```python
from build123d import *

# Parameters (mm, degrees)
F0_W     = 25.4
F0_H     = 25.4
F1_DEPTH = 25.4
F2_R     = 5.08
F2_R_2   = 2.54
F3_DEPTH = 6.35
F4_R     = 1.016
F5_SIZE  = 2.54
F7_D     = 5.1054


with BuildPart() as f1:
    # F0 (on Top) → F1 (new body)
    with BuildSketch(Plane.XY):
        with Locations((12.7, 12.7)):
            Rectangle(F0_W, F0_H)
    extrude(amount=F1_DEPTH)

    # F2 (on face) → F3 (cut)
    with BuildSketch(Plane.XY.offset(25.4)):
        with Locations((12.1342176571, 12.7)):
            Circle(F2_R)
        with Locations((12.1342176571, 12.7)):
            Circle(F2_R_2, mode=Mode.SUBTRACT)
    extrude(amount=-F3_DEPTH, mode=Mode.SUBTRACT)

    # F4
    f4_edges = [f1.edges().sort_by_distance(p)[0] for p in [
        (9.594218, 12.7, 25.4),
        (17.214218, 12.7, 22.225),
        (7.054218, 12.7, 25.4),
        (7.054218, 12.7, 19.05),
    ]]
    fillet(f4_edges, radius=F4_R)

    # F5
    f5_edges = [f1.edges().sort_by_distance(p)[0] for p in [
        (25.4, 12.7, 25.4),
        (25.4, 25.4, 12.7),
        (0, 25.4, 12.7),
        (12.7, 25.4, 0),
        (12.7, 25.4, 25.4),
        (12.7, 0, 25.4),
        (0, 12.7, 25.4),
        (0, 0, 12.7),
        (25.4, 0, 12.7),
        (12.7, 0, 0),
        (0, 12.7, 0),
        (25.4, 12.7, 0),
    ]]
    chamfer(f5_edges, length=F5_SIZE)

    # F7 (through all)
    with Locations(Plane.YZ.offset(25.4)):
        with Locations((19.05, 19.05)):
            Hole(F7_D / 2)


solid = f1.part
```
The model under review builds one solid part; all positions refer to its coordinate system, in mm. A direction names the side the tool comes from. Coordinates: 2 decimals unless noted, no trailing zeros. Order: outer loops, then holes, each group sorted by start corner. A loop starts at its lowest first (then second) coordinate and runs counter-clockwise, first axis right, second up. Notation, with made-up numbers: (73, -25) -> (129, -25) arc R32 cw to (129, 6) -> close; hole circle Ø10 at (68.25, -25). An arc over 180 degrees is marked (long way). Answer in a Markdown table with one row per item. Add a question column.
Item 1: To check wall thickness, follow probe 1 along Z at (x, y) = (17, 19); probe 2 along Y at (x, z) = (13.5, 17.5); probe 3 along Y at (x, z) = (18, 17.75). State the ranges of each line that lie inside material, in increasing order.
Item 2: We need section B-B on x = 21. Write out the cut boundary in (y, z), plus the area to 3 significant figures.
Item 3: We need section A-A on z = 23.5. Write out the cut boundary in (x, y), plus the area to 3 significant figures.
Item 4: We need section C-C on z = 8.5. Write out the cut boundary in (x, y), plus the area to 3 significant figures.
Item 5: Machinability: for faces 1 (the cylindrical face through (11.03, 7.74, 22.26)), 2 (the flat face through (24.15, 24.11, 12.56)), which of the approach directions +Z, -Z, +X, -X, +Y, -Y give a long, thin tool a straight path to every point of the face, cutting with its end or side? Answer none if there is none.
Item 6: We need section D-D on y = 23.75. Write out the cut boundary in (x, z).
Item 7: Clearance check with a flat-ended pin moving along its axis: pin 1 (12 mm diameter, centred on x = 10, y = 17, fed in from +Z). State where the tip first meets the part, or that it passes through.
Item 8: Mouldability with a two-part tool opening along X and no side actions: class faces 3 (the flat face through (10, 11, 19.05)), 4 (the flat face through (1.29, 24.15, 12.56)), 5 (the flat face through (24.11, 12.56, 1.25)) as +X half, -X half, draft (parallel to the pull), parting line (faces both ways), or undercut.
Final values:
| question | item | result |
|---|---|---|
| 1 | probe 1 | z = 0 to 16.5, 21.6 to 25.4 |
| 1 | probe 2 | y = 0 to 17.02, 21.08 to 25.4 |
| 1 | probe 3 | y = 0 to 16.85, 21.25 to 25.4 |
| 2 | outline | (0, 2.54) -> (2.54, 0) -> (22.86, 0) -> (25.4, 2.54) -> (25.4, 22.86) -> (22.86, 25.4) -> (2.54, 25.4) -> (0, 22.86) -> close; hole circle Ø5.11 at (19.05, 19.05) |
| 2 | area | 612 mm2 |
| 3 | outline | (0.64, 2.54) -> (2.54, 0.64) -> (22.86, 0.64) -> (24.76, 2.54) -> (24.76, 22.86) -> (22.86, 24.76) -> (2.54, 24.76) -> (0.64, 22.86) -> close; circle Ø5.08 at (12.13, 12.7); hole circle Ø10.16 at (12.13, 12.7) |
| 3 | area | 514 mm2 |
| 4 | outline | (0, 2.54) -> (2.54, 0) -> (22.86, 0) -> (25.4, 2.54) -> (25.4, 22.86) -> (22.86, 25.4) -> (2.54, 25.4) -> (0, 22.86) -> close |
| 4 | area | 632 mm2 |
| 5 | face 1 | +Z |
| 5 | face 2 | +Z, -Z, +X, +Y |
| 6 | outline | (0.89, 2.54) -> (2.54, 0.89) -> (22.86, 0.89) -> (24.51, 2.54) -> (24.51, 22.86) -> (22.86, 24.51) -> (2.54, 24.51) -> (0.89, 22.86) -> close |
| 7 | pin 1 | stops at z = 25.4 |
| 8 | face 3 | undercut |
| 8 | face 4 | -X half |
| 8 | face 5 | +X half |
